Design review of the part shown in the three views and the two pictorial views. Dimensions are in mm from the part's minimum x, y and z. Round coordinates to 2 decimals unless told otherwise and drop trailing zeros. Write each loop counter-clockwise with the first axis right and the second up, starting at its lowest first coordinate (ties: lowest second). Pieces come first, ordered by that corner, then holes. Notation, with made-up numbers: (89.5, 69) - (95.5, 69) arc R30 cw to (95.5, 95) - close; hole circle Ø6 at (-14, -29). An arc over 180 degrees is marked (long way). One line per item, written item: value. Start each with the question number.
Q1. Mouldability with a two-part tool opening along X and no side actions: class the marked faces 1 and 2 as +X half, -X half, draft (parallel to the pull), parting line (faces both ways), or undercut.
Q2. Add section D-D on z = 4.8. Give the number of separate pieces and of enclosed holes in the cut face.
Q3. Clearance check with flat-ended pins moving along their axes: pin 1 Ø3 at (x, y) = (33, 6) entering from -Z; pin 2 Ø1.5 at (y, z) = (8, 1) entering from +X; pin 3 Ø0.9 at (y, z) = (10, 2) entering from -X; pin 4 Ø2 at (x, z) = (38, 2.5) entering from -Y. State where each tip first meets the part, or that it passes through.
Q4. Add section B-B on x = 10. Write out the cut boundary in (y, z) (1 decimal), and give its area (3 significant figures).
Q5. Add section A-A on x = 33. Write out the cut boundary in (y, z), and give its area (3 significant figures).
Q6. Add section C-C on y = 34. Write out the cut boundary in (x, z).
Q7. For probe 1 along Y at (x, z) = (33, 2.4); probe 2 along X at (y, z) = (46, 2.05) (1 decimal); probe 3 along Z at (x, y) = (59.5, 41.5), list the stretches that pass through material, from the lowest coordinate up.
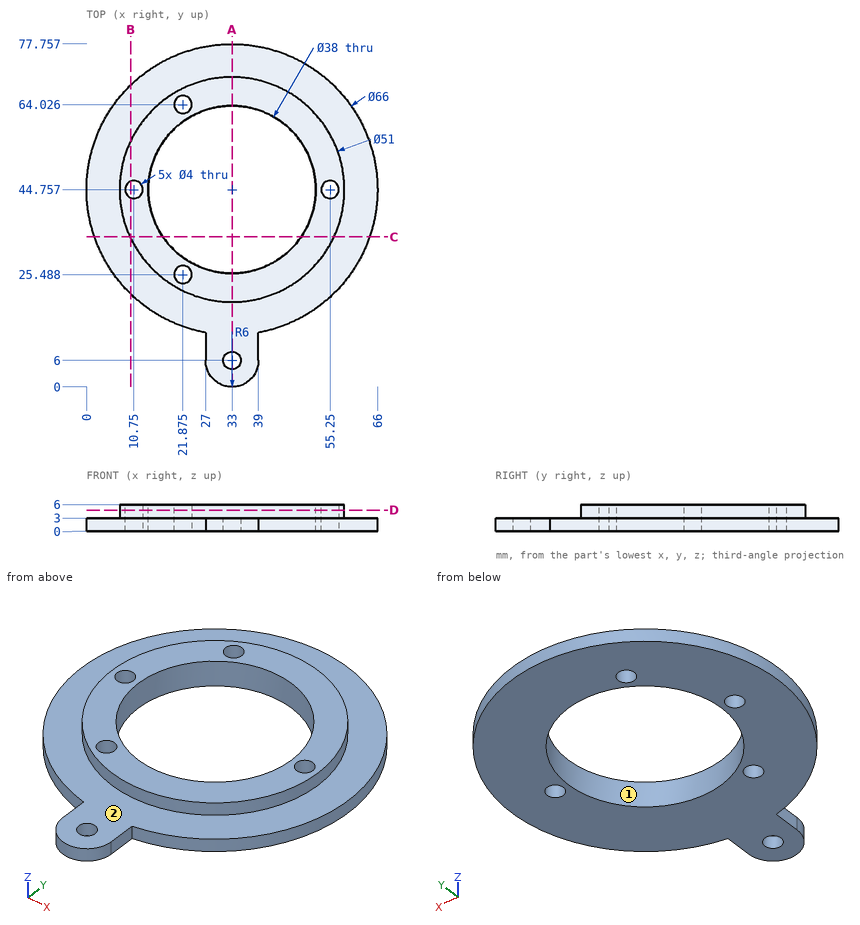
Result set:
1. face 1: undercut
1. face 2: draft
2. separate pieces: 1
2. enclosed holes: 5
3. pin 1: passes through
3. pin 2: stops at x = 39
3. pin 3: stops at x = 27
3. pin 4: stops at y = 1.53
4. outline: (21.1, 0) - (42.9, 0) - (42.9, 6) - (33.7, 6) - (33.7, 3) - (21.1, 3) - close; (46.6, 0) - (68.4, 0) - (68.4, 3) - (55.8, 3) - (55.8, 6) - (46.6, 6) - close
4. area: 186 mm^2
5. outline: (0, 0) - (4, 0) - (4, 3) - (0, 3) - close; (8, 0) - (25.76, 0) - (25.76, 6) - (19.26, 6) - (19.26, 3) - (8, 3) - close; (63.76, 0) - (77.76, 0) - (77.76, 3) - (70.26, 3) - (70.26, 6) - (63.76, 6) - close
5. area: 146 mm^2
6. outline: (1.8, 0) - (17.34, 0) - (17.34, 6) - (9.88, 6) - (9.88, 3) - (1.8, 3) - close; (48.66, 0) - (64.2, 0) - (64.2, 3) - (56.12, 3) - (56.12, 6) - (48.66, 6) - close
7. probe 1: y = 0 to 4, 8 to 25.76, 63.76 to 77.76
7. probe 2: x = 0 to 9.2, 12.3 to 14, 52 to 53.7, 56.8 to 66
7. probe 3: z = 0 to 3
